Could you check a few things on this drawing? It's one solid part, dimensions in mm from its lowest x, y, z. Coordinates: 2 decimals unless noted, no trailing zeros. Loops run counter-clockwise (first coordinate to the right, second up) from the corner with the lowest first, then second, coordinate; pieces in that order, holes last. Notation, with made-up numbers: M -39.5,42.25 L -27.5,42.25 A10 cw -27.5,50.25 Z; hole C 36,-40 d8. An arc over 180 degrees is marked long. Answer as a JSON object with one key per item and string values. Group by question number.
Item 1: I'm going to push a flat-ended pin straight in: pin 1 Ø3 at (x, y) = (112.5, 2.5) entering from +Z. Where does the tip first touch, or does it pass through?
Item 2: If I drill on line 1 (Y direction, x = 2.5, z = 0.6); line 2 (X direction, y = 2.5, z = 1.1), over which ranges is the centre line in solid material (lowest first)?
Item 3: Suppose I cut it at A-A (y = 37.5). Write out the boundary of the cut face in (x, z).
Item 4: Suppose I cut it at B-B (x = 112.5). Write out the boundary of the cut face in (y, z), then the cut area to 3 significant figures.
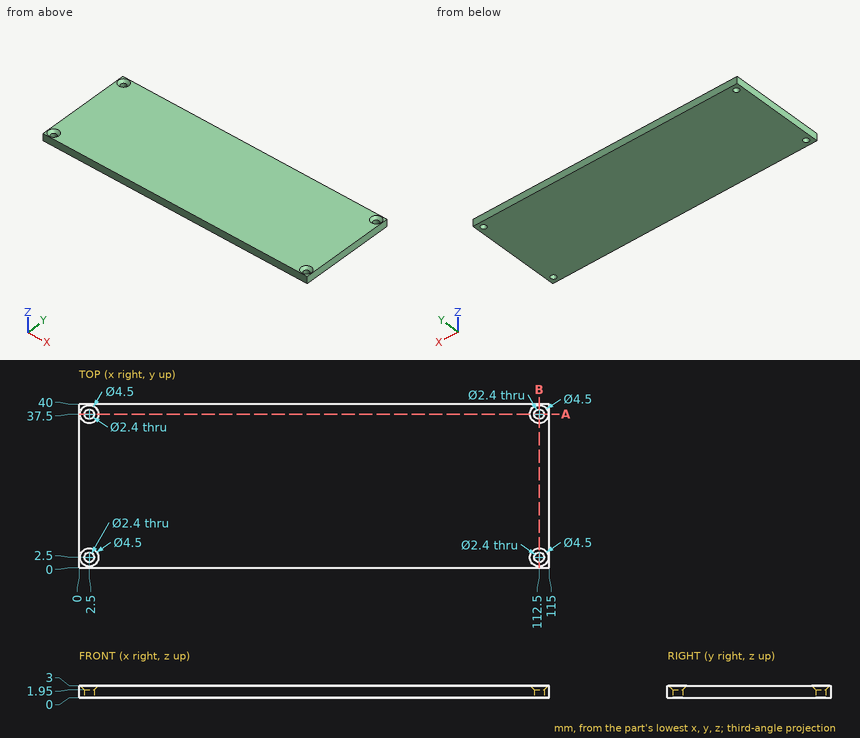
From the geometry:
{
 "1": {"pin 1": "z = 2.25"},
 "2": {"line 1": "0 to 1.3, 3.7 to 36.3, 38.7 to 40", "line 2": "0 to 1.3, 3.7 to 111.3, 113.7 to 115"},
 "3": {"outline": "M 0,0 L 1.3,0 L 1.3,1.95 L 0.25,3 L 0,3 Z; M 3.7,0 L 111.3,0 L 111.3,1.95 L 110.25,3 L 4.75,3 L 3.7,1.95 Z; M 113.7,0 L 115,0 L 115,3 L 114.75,3 L 113.7,1.95 Z"},
 "4": {"outline": "M 0,0 L 1.3,0 L 1.3,1.95 L 0.25,3 L 0,3 Z; M 3.7,0 L 36.3,0 L 36.3,1.95 L 35.25,3 L 4.75,3 L 3.7,1.95 Z; M 38.7,0 L 40,0 L 40,3 L 39.75,3 L 38.7,1.95 Z", "area": "103 mm2"}
}
